Input: dimensioned drawing with shaded views. Units: mm. Origin: part minimum x, y, z. A direction names the side the tool comes from. Round coordinates to 2 decimals unless told otherwise and drop trailing zeros. Order: outer loops, then holes, each group sorted by start corner. A loop starts at its lowest first (then second) coordinate and runs counter-clockwise, first axis right, second up. Notation, with made-up numbers: M -31,-6.5 L -6,-6.5 A8 ccw -6,8.5 Z; hole C -29.5,-31.75 d10. An arc over 180 degrees is marked long. One line per question, with ' | ' between items.
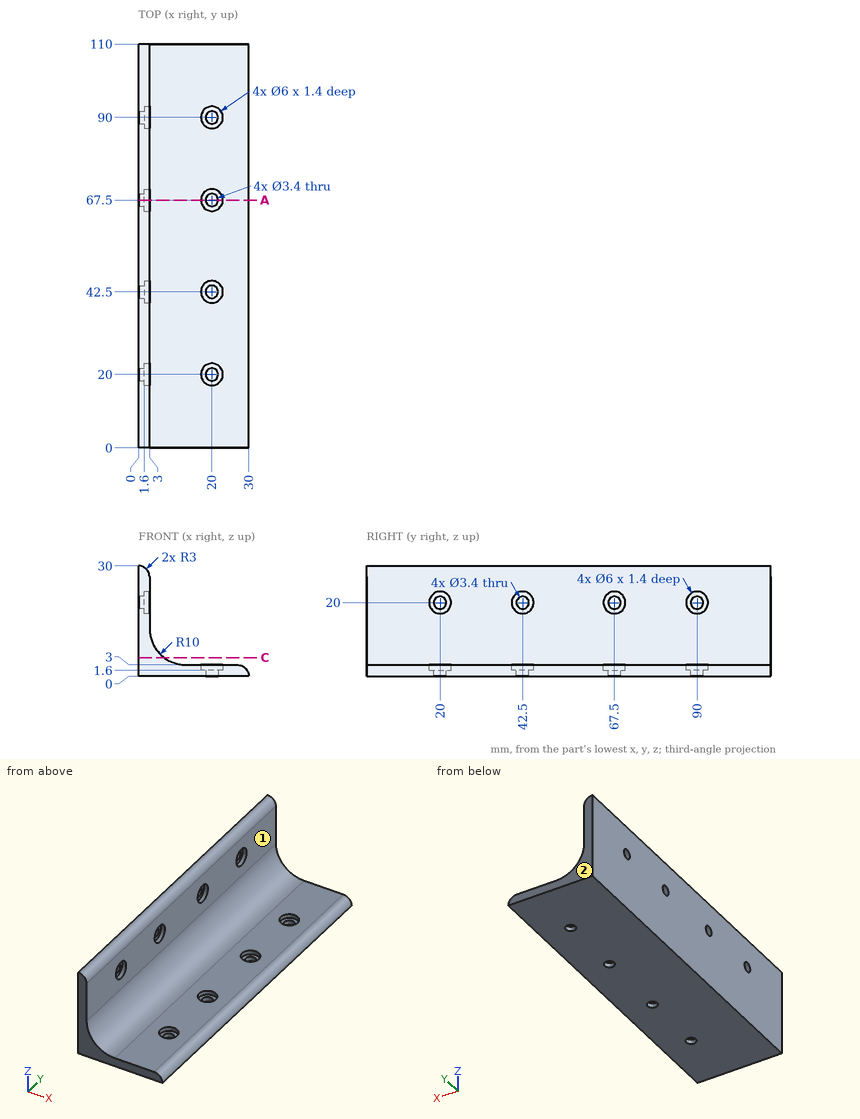
Item 1: Access query for the marked faces 1 and 2. Directions: +Z, -Z, +X, -X, +Y, -Y. A direction counts if a zero-diameter tool reaches every point of the face in a straight line with its end or side. Return the directions, or none.
Report:
face 1: +Z, +X, +Y, -Y | face 2: +Z, -Z, +X, -X, +Y
Item 2: Line query: line 1 along Y through (x, z) = (2.2, 20); line 2 along Y through (x, z) = (0.7, 20); line 3 along Z through (x, y) = (27.25, 99). Output: solid intervals per line, ascending. Write a range as from..to.
Report:
line 1: 0..17, 23..39.5, 45.5..64.5, 70.5..87, 93..110 | line 2: 0..18.3, 21.7..40.8, 44.2..65.8, 69.2..88.3, 91.7..110 | line 3: 0..2.99
Item 3: Section query C-C, the plane z = 5. Return loops of the section in (x, y), plus the area to 3 significant figures.
Report:
outline: M 0,0 L 7,0 L 7,110 L 0,110 Z | area: 770 mm²
Item 4: Section query A-A, the plane y = 67.5. Give the number of separate pieces and of enclosed holes in the cut face, plus the area to 3 significant figures.
Report:
separate pieces: 3 | enclosed holes: 0 | area: 161 mm²
Item 5: First-contact query: pin 1 (8 mm diameter, centred on y = 80, z = 27, fed in from +X); pin 2 (1 mm diameter, centred on x = 10.5, y = 59, fed in from +Z); pin 3 (8 mm diameter, centred on y = 82, z = 14, fed in from +X); pin 4 (2.5 mm diameter, centred on x = 20, y = 90, fed in from -Z). Flat tips, straight axial feed; report the tip coordinate or a pass-through.
Report:
pin 1: x = 3 | pin 2: z = 3.46 | pin 3: x = 3.46 | pin 4: through
